Build history of the part. All positions in model axes, mm. Face numbers are marked on the shaded views. Round coordinates to 2 decimals unless told otherwise and drop trailing zeros. Write each loop counter-clockwise with the first axis right and the second up, starting at its lowest first coordinate (ties: lowest second). Pieces come first, ordered by that corner, then holes. Notation, with made-up numbers: (-16.75, 53) -> (4.25, 53) arc R29 cw to (4.25, 92) -> close; hole circle Ø6 at (-28, -12). An arc over 180 degrees is marked (long way). Answer as CSV lines item,"result".
from build123d import *

# Parameters (mm, degrees)
SKETCH_1_W          = 150
SKETCH_1_H          = 70
EXTRUDE_1_DEPTH     = 3
FILLET_1_R          = 5
SKETCH_2_R          = 1.5
CUT_EXTRUDE_1_DEPTH = 3
SKETCH_3_R          = 2.5
CUT_EXTRUDE_2_DEPTH = 2
SKETCH_4_W          = 3
SKETCH_4_H          = 30
SKETCH_4_W_2        = 60
SKETCH_4_H_2        = 3
EXTRUDE_2_DEPTH     = 2


with BuildPart() as part:
    # Эскиз1 → Бобышка-Вытянуть1 (new body)
    with BuildSketch(Plane(origin=(0, 0, 0), x_dir=(1, 0, 0), z_dir=(0, 1, 0))):
        Rectangle(SKETCH_1_W, SKETCH_1_H)
    extrude(amount=EXTRUDE_1_DEPTH)

    # Скругление1
    fillet_1_edges = [part.edges().sort_by_distance(p)[0] for p in [
        (75, 1.5, -35),
        (75, 1.5, 35),
        (-75, 1.5, 35),
        (-75, 1.5, -35),
    ]]
    fillet(fillet_1_edges, radius=FILLET_1_R)

    # Эскиз2 → Вырез-Вытянуть1 (cut)
    with BuildSketch(Plane(origin=(0, 3, 0), x_dir=(1, 0, 0), z_dir=(0, 1, 0))):
        with Locations(Location((-70, 30, 0), (0, 0, 270))):
            Circle(SKETCH_2_R)
        with Locations(Location((70, 30, 0), (0, 0, 270))):
            Circle(SKETCH_2_R)
        with Locations(Location((70, -30, 0), (0, 0, 270))):
            Circle(SKETCH_2_R)
        with Locations(Location((-70, -30, 0), (0, 0, 270))):
            Circle(SKETCH_2_R)
    extrude(amount=-CUT_EXTRUDE_1_DEPTH, mode=Mode.SUBTRACT)

    # Эскиз3 → Вырез-Вытянуть2 (cut)
    with BuildSketch(Plane(origin=(0, 3, 0), x_dir=(1, 0, 0), z_dir=(0, 1, 0))):
        with Locations(Location((-70, 30, 0), (0, 0, 270))):
            Circle(SKETCH_3_R)
        with Locations(Location((70, 30, 0), (0, 0, 270))):
            Circle(SKETCH_3_R)
        with Locations(Location((70, -30, 0), (0, 0, 270))):
            Circle(SKETCH_3_R)
        with Locations(Location((-70, -30, 0), (0, 0, 270))):
            Circle(SKETCH_3_R)
    extrude(amount=-CUT_EXTRUDE_2_DEPTH, mode=Mode.SUBTRACT)

    # Эскиз4 → Бобышка-Вытянуть2 (add)
    with BuildSketch(Plane.XZ):
        with Locations((-70.5, 0)):
            Rectangle(SKETCH_4_W, SKETCH_4_H)
        with Locations((0, -30.5)):
            Rectangle(SKETCH_4_W_2, SKETCH_4_H_2)
        with Locations((70.5, 0)):
            Rectangle(SKETCH_4_W, SKETCH_4_H)
        with Locations((0, 30.5)):
            Rectangle(SKETCH_4_W_2, SKETCH_4_H_2)
    extrude(amount=EXTRUDE_2_DEPTH)


solid = part.part
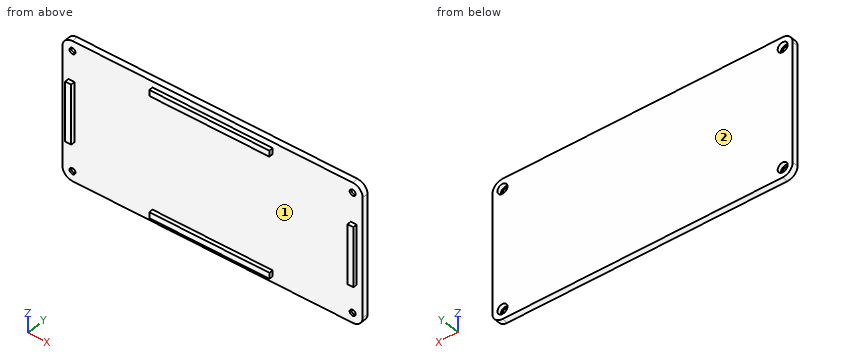
1. Probe line 1 along Z through (x, y) = (-70, 0.5); line 2 along X through (y, z) = (2.1, -30); line 3 along Z through (x, y) = (-25, -0.7). List the from-to ranges inside material, lowest first.
Results found:
line 1,"z = -35 to -31.5, -28.5 to 28.5, 31.5 to 35"
line 2,"x = -75 to -72.5, -67.5 to 67.5, 72.5 to 75"
line 3,"z = -32 to -29, 29 to 32"
2. Mould opens along Z. For the marked faces 1 and 2 say: +Z half, -Z half, draft (parallel to the pull), parting line (faces both ways), or undercut.
Results found:
face 1,"undercut"
face 2,"draft"
3. Cut at D-D, the plane x = -32. Write the cut outline in (y, z).
Results found:
outline,"(0, -35) -> (3, -35) -> (3, 35) -> (0, 35) -> close"
4. Cut at B-B, the plane x = -1. Write the cut outline in (y, z), then the cut area to 3 significant figures.
Results found:
outline,"(-2, -32) -> (0, -32) -> (0, -35) -> (3, -35) -> (3, 35) -> (0, 35) -> (0, 32) -> (-2, 32) -> (-2, 29) -> (0, 29) -> (0, -29) -> (-2, -29) -> close"
area,"222 mm2"
5. Cut at A-A, the plane y = -1.15. Write the cut outline in (x, z).
Results found:
outline,"(-72, -15) -> (-69, -15) -> (-69, 15) -> (-72, 15) -> close; (-30, -32) -> (30, -32) -> (30, -29) -> (-30, -29) -> close; (-30, 29) -> (30, 29) -> (30, 32) -> (-30, 32) -> close; (69, -15) -> (72, -15) -> (72, 15) -> (69, 15) -> close"
6. Cut at C-C, the plane z = 18.5. Write the cut outline in (x, y), then the cut area to 3 significant figures.
Results found:
outline,"(-75, 0) -> (75, 0) -> (75, 3) -> (-75, 3) -> close"
area,"450 mm2"
7. Drop flat-ended pins along their axis: pin 1 Ø21 at (x, z) = (-0.5, -15.5) entering from -Y; pin 2 Ø1.5 at (x, z) = (71, 30.5) entering from +Y; pin 3 Ø2 at (y, z) = (-1.5, 2.5) entering from -X. Give the stop position or say it passes through.
Results found:
pin 1,"stops at y = 0"
pin 2,"stops at y = 1"
pin 3,"stops at x = -72"
